Here's how the part is built. I have some questions about the finished solid (model axes, mm). A direction names the side the tool comes from. Round coordinates to 2 decimals unless told otherwise and drop trailing zeros. Loops run counter-clockwise (first coordinate to the right, second up) from the corner with the lowest first, then second, coordinate; pieces in that order, holes last. Notation, with made-up numbers: (68.25, 34) - (100.25, 34) arc R18 ccw to (100.25, 47) - close; hole circle Ø2 at (-0.5, -29). An arc over 180 degrees is marked (long way). Answer as a JSON object with one key per item and string values. Group by question number.
1) I want a section at B-B, the plane z = 16. Please give me the cut outline in (x, y), then the cut area to 3 significant figures.
2) I want a section at C-C, the plane x = -15.5. Please give me the cut outline in (y, z).
3) If we mould it in two halves opening along X, with no side actions, what happens to faces 4 (the face through (11.9, 12, 0)), 5 (the face through (-29.8, 0, 0)), 6 (the face through (11.9, -12, 0)), 7 (the face through (24, -14.9, 0))? For each: pulls with the +X half, pulls with the -X half, needs draft (parallel to the pull), parting line crosses it, or undercut.
4) I want a section at A-A, the plane y = 11.75. Please give me the cut outline in (x, z).
5) Will these pins go through, and if not, where does the flat tip stop? P1, Ø1.8, axis at x = -16, z = 8.5, coming from the -Y side; P2, Ø5, axis at x = 15, z = -17.5, coming from the +Y side.
6) If I drill on line 1 along X through (y, z) = (13.25, 13.5); line 2 along Y through (x, z) = (-15, -18), over which ranges is the centre line in solid material (lowest first)? Write a range as [from, to].
7) Which directions (+Z, -Z, +X, -X, +Y, -Y) give clear straight access to the entire face, cutting with the end or side of a thin tool? Please do faces 1 (the face through (24, 14.9, 0)), 2 (the face through (-11.9, 12, 0)), 3 (the face through (-17.9, -12, 0)).
Autodesk Inventor part; units mm, degrees
ref_plane "YZ Plane" through (0, 0, 0) normal (1, 0, 0) x (0, 1, 0)
ref_plane "XZ Plane" through (0, 0, 0) normal (0, 1, 0) x (-1, 0, 0)
ref_plane "XY Plane" through (0, 0, 0) normal (0, 0, 1) x (1, 0, 0)
sketch "Sketch1" plane through (0, 0, 0) normal (0, 1, 0) x (-1, 0, 0)
  line L0 (-29.8, 35.3) -> (29.8, 35.3)
  line L1 (29.8, 35.3) -> (29.8, -35.3)
  line L2 (29.8, -35.3) -> (-29.8, -35.3)
  line L3 (-29.8, -35.3) -> (-29.8, 35.3)
  line L4 (-29.8, 35.3) -> (29.8, -35.3) construction
  line L5 (29.8, 35.3) -> (-29.8, -35.3) construction
  point P0 (0, 0)
  dimension "d0" = 70.6
  dimension "d1" = 59.6
extrude "Extrusion1" add sketch "Sketch1" along normal mid plane 29.8
sketch "Sketch2" plane through (0, 14.9, 0) normal (0, 1, 0) x (1, 0, 0)
  line L0 (-29.8, -35.3) -> (29.8, -35.3)
  line L1 (29.8, 35.3) -> (-29.8, 35.3)
  line L2 (-17.9, -35.3) -> (-11.9, -35.3)
  line L3 (-11.9, -35.3) -> (-11.9, 35.3)
  line L4 (-11.9, 35.3) -> (-17.9, 35.3)
  line L5 (-17.9, 35.3) -> (-17.9, -35.3)
  line L6 (11.9, -35.3) -> (17.9, -35.3)
  line L7 (17.9, -35.3) -> (17.9, 35.3)
  line L8 (17.9, 35.3) -> (11.9, 35.3)
  line L9 (11.9, 35.3) -> (11.9, -35.3)
  line L10 (-29.8, 35.3) -> (-29.8, -35.3)
  line L11 (0, -35.3) -> (0, 35.3) construction
  point P0 (0, 0)
  dimension "d4" = 6
  dimension "d5" = 11.9
extrude "Extrusion2" cut sketch "Sketch2" against normal blind 6 contours L5 L1 L3 L0 | L9 L1 L7 L0
mirror "Mirror1" about plane through (0, 0, 0) normal (0, 1, 0) of "Extrusion2"
properties part number "Linear Rail Carriage"
Outcome:
{
 "1": {"outline": "(-29.8, -14.9) - (-17.9, -14.9) - (-17.9, -8.9) - (-11.9, -8.9) - (-11.9, -14.9) - (11.9, -14.9) - (11.9, -8.9) - (17.9, -8.9) - (17.9, -14.9) - (29.8, -14.9) - (29.8, 14.9) - (17.9, 14.9) - (17.9, 8.9) - (11.9, 8.9) - (11.9, 14.9) - (-11.9, 14.9) - (-11.9, 8.9) - (-17.9, 8.9) - (-17.9, 14.9) - (-29.8, 14.9) - close", "area": "1,630 mm^2"},
 "2": {"outline": "(-8.9, -35.3) - (8.9, -35.3) - (8.9, 35.3) - (-8.9, 35.3) - close"},
 "3": {"face 4": "undercut", "face 5": "pulls with the -X half", "face 6": "undercut", "face 7": "needs draft"},
 "4": {"outline": "(-29.8, -35.3) - (-17.9, -35.3) - (-17.9, 35.3) - (-29.8, 35.3) - close; (-11.9, -35.3) - (11.9, -35.3) - (11.9, 35.3) - (-11.9, 35.3) - close; (17.9, -35.3) - (29.8, -35.3) - (29.8, 35.3) - (17.9, 35.3) - close"},
 "5": {"P1": "y = -8.9", "P2": "y = 8.9"},
 "6": {"line 1": "[-29.8, -17.9], [-11.9, 11.9], [17.9, 29.8]", "line 2": "[-8.9, 8.9]"},
 "7": {"face 1": "+Z, -Z, +X, -X, +Y", "face 2": "+Z, -Z, +Y", "face 3": "+Z, -Z, -Y"}
}
